Work out the finished part from the listing and answer in its coordinate system (mm). Face numbers are marked on the shaded views. A direction names the side the tool comes from. Coordinates: 2 decimals unless noted, no trailing zeros. Order: outer loops, then holes, each group sorted by start corner. A loop starts at its lowest first (then second) coordinate and runs counter-clockwise, first axis right, second up. Notation, with made-up numbers: M -40,67 L -8,67 A20 cw -8,93 Z; hole C 75,-4.75 d7. An arc over 180 degrees is marked long. Use a Markdown table: item, result.
from build123d import *

# Parameters (mm, degrees)
BOSS_EXTRUDE1_DEPTH   = 30
CUT_EXTRUDE1_DEPTH    = 5
FILLET1_R             = 5
CHAMFER1_SIZE         = 1
M3X0_5_TAPPED_HOLE1_D = 2.5


with BuildPart() as part:
    # Sketch1 → Boss-Extrude1 (new, symmetric)
    with BuildSketch(Plane(origin=(0, 0, 0), x_dir=(0, 0, -1), z_dir=(1, 0, 0))):
        Polygon((-17.5, 10), (17.5, 10), (17.5, 0), (4, 0), (4, -3), (-4, -3), (-4, 0), (-17.5, 0), align=None)
    extrude(amount=BOSS_EXTRUDE1_DEPTH, both=True)

    # Sketch3 → CSK for M6 Flat Head Machine Screw1 (revolve, cut)
    with BuildSketch(Plane(origin=(0, 10, 0), x_dir=(0, 0, 1), z_dir=(1, 0, 0))):
        Polygon((0, 0), (0, 13), (3.3, 13), (3.3, 8), (6.3, 5), (6.3, 0), align=None)
    revolve(axis=Axis((0, 16.35, 0), (0, -1, 0)), mode=Mode.SUBTRACT)

    # Sketch4 → Cut-Extrude1 (cut, symmetric)
    with BuildSketch(Plane(origin=(20, 0, 0), x_dir=(0, 0, -1), z_dir=(1, 0, 0))):
        with BuildLine():
            Line((-15, 10), (-10, 10))
            ThreePointArc((-10, 10), (-7.5, 7.5), (-5, 10))
            Line((-5, 10), (0, 10))
            ThreePointArc((0, 10), (-7.5, 2.5), (-15, 10))
        make_face()
    cut_extrude1 = extrude(amount=CUT_EXTRUDE1_DEPTH, both=True, mode=Mode.SUBTRACT)

    # Mirror1: Cut-Extrude1 across plane
    add(cut_extrude1.mirror(Plane(origin=(0, 0, 0), x_dir=(0, 0, 1), z_dir=(1, 0, 0))), mode=Mode.SUBTRACT)

    # Fillet1
    fillet1_edges = [part.edges().sort_by_distance(p)[0] for p in [
        (-30, 5, 17.5),
        (30, 5, -17.5),
        (30, 5, 17.5),
        (-30, 5, -17.5),
    ]]
    fillet(fillet1_edges, radius=FILLET1_R)

    # Chamfer1
    # the kernel refuses this chamfer: 1 mm, written as the material it takes off along each edge
    with BuildSketch(Plane(origin=(-30, -5.571682988, 4), x_dir=(-0.027495876610585623, 0, -0.9996219169112968), z_dir=(0, 1, 0)), Plane(origin=(-30, 0, -4), x_dir=(-0.027495876610585623, 0, 0.9996219169112968), z_dir=(0, -1, 0))) as chamfer1_piece_1:
        Polygon((CHAMFER1_SIZE * 0.999621916911, -CHAMFER1_SIZE * 0.0274958766106), (-CHAMFER1_SIZE * 0.0274958766106, -CHAMFER1_SIZE * 0.999621916911), (0, 0), align=None)
    extrude(amount=5.571682988, mode=Mode.SUBTRACT)
    with BuildSketch(Plane(origin=(30, -5.571682988, 4), x_dir=(0.027495876610585623, 0, -0.9996219169112968), z_dir=(0, 1, 0)), Plane(origin=(30, 0, -4), x_dir=(0.027495876610585623, 0, 0.9996219169112968), z_dir=(0, -1, 0))) as chamfer1_piece_2:
        Polygon((CHAMFER1_SIZE * 0.999621916911, CHAMFER1_SIZE * 0.0274958766106), (-CHAMFER1_SIZE * 0.0274958766106, CHAMFER1_SIZE * 0.999621916911), (0, 0), align=None)
    extrude(amount=5.571682988, mode=Mode.SUBTRACT)
    with BuildSketch(Plane(origin=(32.571682988, -3, -4), x_dir=(0, 0.9996219169112968, -0.027495876610586494), z_dir=(-1, 0, 0))) as chamfer1_piece_3:
        Polygon((CHAMFER1_SIZE * 0.999621916911, -CHAMFER1_SIZE * 0.0274958766106), (-CHAMFER1_SIZE * 0.0274958766106, -CHAMFER1_SIZE * 0.999621916911), (0, 0), align=None)
    extrude(amount=65.143365976, mode=Mode.SUBTRACT)
    with BuildSketch(Plane(origin=(32.571682988, -3, 4), x_dir=(0, 0.9996219169112968, 0.027495876610586494), z_dir=(-1, 0, 0))) as chamfer1_piece_4:
        Polygon((CHAMFER1_SIZE * 0.999621916911, CHAMFER1_SIZE * 0.0274958766106), (-CHAMFER1_SIZE * 0.0274958766106, CHAMFER1_SIZE * 0.999621916911), (0, 0), align=None)
    extrude(amount=65.143365976, mode=Mode.SUBTRACT)
    with BuildSketch(Plane(origin=(30, 0, -12.5), x_dir=(0.027495876610585623, 0.9996219169112968, 0), z_dir=(0, 0, 1)), Plane(origin=(30, 0, 4), x_dir=(0.02749587661058563, 0.9996219169112968, 0), z_dir=(0, 0, 1))) as chamfer1_piece_5:
        Polygon((CHAMFER1_SIZE * 0.999621916911, CHAMFER1_SIZE * 0.0274958766106), (-CHAMFER1_SIZE * 0.0274958766106, CHAMFER1_SIZE * 0.999621916911), (0, 0), align=None)
    extrude(amount=8.5, mode=Mode.SUBTRACT)
    with BuildSketch(Plane(origin=(-30, 0, 4), x_dir=(-0.02749587661058563, 0.9996219169112968, 0), z_dir=(0, 0, 1)), Plane(origin=(-30, 0, -12.5), x_dir=(-0.027495876610585623, 0.9996219169112968, 0), z_dir=(0, 0, 1))) as chamfer1_piece_6:
        Polygon((CHAMFER1_SIZE * 0.999621916911, -CHAMFER1_SIZE * 0.0274958766106), (-CHAMFER1_SIZE * 0.0274958766106, -CHAMFER1_SIZE * 0.999621916911), (0, 0), align=None)
    extrude(amount=8.5, mode=Mode.SUBTRACT)
    with BuildSketch(Plane(origin=(-25, 0, 17.5), x_dir=(0, 0.9996219169112968, 0.02749587661058563), z_dir=(1, 0, 0)), Plane(origin=(25, 0, -17.5), x_dir=(0, 0.9996219169112968, -0.027495876610585623), z_dir=(-1, 0, 0))) as chamfer1_piece_7:
        Polygon((CHAMFER1_SIZE * 0.999621916911, -CHAMFER1_SIZE * 0.0274958766106), (-CHAMFER1_SIZE * 0.0274958766106, -CHAMFER1_SIZE * 0.999621916911), (0, 0), align=None)
    extrude(amount=50, mode=Mode.SUBTRACT)
    with BuildSketch(Plane(origin=(-25, 0, 12.5), x_dir=(0, 0, 1), z_dir=(1, 0, 0))) as chamfer1_piece_8:
        Polygon((5, -CHAMFER1_SIZE), (5 - CHAMFER1_SIZE, 0), (5, 0), align=None)
    revolve(axis=Axis((-25, 0, 12.5), (0, -1, 0)), revolution_arc=90, mode=Mode.SUBTRACT)
    with BuildSketch(Plane(origin=(25, 0, 12.5), x_dir=(0, 0, 1), z_dir=(-1, 0, 0))) as chamfer1_piece_9:
        Polygon((5, CHAMFER1_SIZE), (5 - CHAMFER1_SIZE, 0), (5, 0), align=None)
    revolve(axis=Axis((25, 0, 12.5), (0, 1, 0)), revolution_arc=90, mode=Mode.SUBTRACT)
    with BuildSketch(Plane(origin=(-25, 0, -12.5), x_dir=(-1, 0, 0), z_dir=(0, 0, 1))) as chamfer1_piece_10:
        Polygon((5, -CHAMFER1_SIZE), (5 - CHAMFER1_SIZE, 0), (5, 0), align=None)
    revolve(axis=Axis((-25, 0, -12.5), (0, -1, 0)), revolution_arc=90, mode=Mode.SUBTRACT)
    with BuildSketch(Plane(origin=(25, 0, -12.5), x_dir=(1, 0, 0), z_dir=(0, 0, 1))) as chamfer1_piece_11:
        Polygon((5, CHAMFER1_SIZE), (5 - CHAMFER1_SIZE, 0), (5, 0), align=None)
    revolve(axis=Axis((25, 0, -12.5), (0, 1, 0)), revolution_arc=90, mode=Mode.SUBTRACT)
    with BuildSketch(Plane(origin=(-30, 0, 1.428317012), x_dir=(-0.02749587661058563, 0.9996219169112968, 0), z_dir=(0, 0, 1))) as chamfer1_piece_12a_section:
        Polygon((CHAMFER1_SIZE * 0.999621916911, -CHAMFER1_SIZE * 0.0274958766106), (-CHAMFER1_SIZE * 0.0274958766106, -CHAMFER1_SIZE * 0.999621916911), (0, 0), align=None)
    chamfer1_piece_12a = extrude(amount=11.071682988, mode=Mode.PRIVATE)
    chamfer1_piece_12a = split(chamfer1_piece_12a, bisect_by=Plane(origin=(-29.670206373, 0.329793627, 4), z_dir=(0, 0, -1)), keep=Keep.TOP, mode=Mode.PRIVATE)
    with BuildSketch(Plane(origin=(-30, -5.571682988, 4), x_dir=(-0.027495876610585623, 0, -0.9996219169112968), z_dir=(0, 1, 0))) as chamfer1_piece_12b_section:
        Polygon((CHAMFER1_SIZE * 0.999621916911, -CHAMFER1_SIZE * 0.0274958766106), (-CHAMFER1_SIZE * 0.0274958766106, -CHAMFER1_SIZE * 0.999621916911), (0, 0), align=None)
    chamfer1_piece_12b = extrude(amount=8.143365976, mode=Mode.PRIVATE)
    chamfer1_piece_12b = split(chamfer1_piece_12b, bisect_by=Plane(origin=(-29.670206373, 0, 3.670206373), z_dir=(0, 1, 0)), keep=Keep.TOP, mode=Mode.PRIVATE)
    chamfer1_piece_12 = chamfer1_piece_12a & chamfer1_piece_12b
    add(chamfer1_piece_12, mode=Mode.SUBTRACT)
    with BuildSketch(Plane(origin=(30, 0, 1.428317012), x_dir=(0.02749587661058563, 0.9996219169112968, 0), z_dir=(0, 0, 1))) as chamfer1_piece_13a_section:
        Polygon((CHAMFER1_SIZE * 0.999621916911, CHAMFER1_SIZE * 0.0274958766106), (-CHAMFER1_SIZE * 0.0274958766106, CHAMFER1_SIZE * 0.999621916911), (0, 0), align=None)
    chamfer1_piece_13a = extrude(amount=11.071682988, mode=Mode.PRIVATE)
    chamfer1_piece_13a = split(chamfer1_piece_13a, bisect_by=Plane(origin=(29.670206373, 0.329793627, 4), z_dir=(0, 0, -1)), keep=Keep.TOP, mode=Mode.PRIVATE)
    with BuildSketch(Plane(origin=(30, -5.571682988, 4), x_dir=(0.027495876610585623, 0, -0.9996219169112968), z_dir=(0, 1, 0))) as chamfer1_piece_13b_section:
        Polygon((CHAMFER1_SIZE * 0.999621916911, CHAMFER1_SIZE * 0.0274958766106), (-CHAMFER1_SIZE * 0.0274958766106, CHAMFER1_SIZE * 0.999621916911), (0, 0), align=None)
    chamfer1_piece_13b = extrude(amount=8.143365976, mode=Mode.PRIVATE)
    chamfer1_piece_13b = split(chamfer1_piece_13b, bisect_by=Plane(origin=(29.670206373, 0, 3.670206373), z_dir=(0, 1, 0)), keep=Keep.TOP, mode=Mode.PRIVATE)
    chamfer1_piece_13 = chamfer1_piece_13a & chamfer1_piece_13b
    add(chamfer1_piece_13, mode=Mode.SUBTRACT)
    with BuildSketch(Plane(origin=(30, 0, -12.5), x_dir=(0.027495876610585623, 0.9996219169112968, 0), z_dir=(0, 0, 1))) as chamfer1_piece_14a_section:
        Polygon((CHAMFER1_SIZE * 0.999621916911, CHAMFER1_SIZE * 0.0274958766106), (-CHAMFER1_SIZE * 0.0274958766106, CHAMFER1_SIZE * 0.999621916911), (0, 0), align=None)
    chamfer1_piece_14a = extrude(amount=11.071682988, mode=Mode.PRIVATE)
    chamfer1_piece_14a = split(chamfer1_piece_14a, bisect_by=Plane(origin=(29.670206373, 0.329793627, -4), z_dir=(0, 0, 1)), keep=Keep.TOP, mode=Mode.PRIVATE)
    with BuildSketch(Plane(origin=(30, 2.571682988, -4), x_dir=(0.027495876610585623, 0, 0.9996219169112968), z_dir=(0, -1, 0))) as chamfer1_piece_14b_section:
        Polygon((CHAMFER1_SIZE * 0.999621916911, CHAMFER1_SIZE * 0.0274958766106), (-CHAMFER1_SIZE * 0.0274958766106, CHAMFER1_SIZE * 0.999621916911), (0, 0), align=None)
    chamfer1_piece_14b = extrude(amount=8.143365976, mode=Mode.PRIVATE)
    chamfer1_piece_14b = split(chamfer1_piece_14b, bisect_by=Plane(origin=(29.670206373, 0, -3.670206373), z_dir=(0, 1, 0)), keep=Keep.TOP, mode=Mode.PRIVATE)
    chamfer1_piece_14 = chamfer1_piece_14a & chamfer1_piece_14b
    add(chamfer1_piece_14, mode=Mode.SUBTRACT)
    with BuildSketch(Plane(origin=(-30, 0, -12.5), x_dir=(-0.027495876610585623, 0.9996219169112968, 0), z_dir=(0, 0, 1))) as chamfer1_piece_15a_section:
        Polygon((CHAMFER1_SIZE * 0.999621916911, -CHAMFER1_SIZE * 0.0274958766106), (-CHAMFER1_SIZE * 0.0274958766106, -CHAMFER1_SIZE * 0.999621916911), (0, 0), align=None)
    chamfer1_piece_15a = extrude(amount=11.071682988, mode=Mode.PRIVATE)
    chamfer1_piece_15a = split(chamfer1_piece_15a, bisect_by=Plane(origin=(-29.670206373, 0.329793627, -4), z_dir=(0, 0, 1)), keep=Keep.TOP, mode=Mode.PRIVATE)
    with BuildSketch(Plane(origin=(-30, 2.571682988, -4), x_dir=(-0.027495876610585623, 0, 0.9996219169112968), z_dir=(0, -1, 0))) as chamfer1_piece_15b_section:
        Polygon((CHAMFER1_SIZE * 0.999621916911, -CHAMFER1_SIZE * 0.0274958766106), (-CHAMFER1_SIZE * 0.0274958766106, -CHAMFER1_SIZE * 0.999621916911), (0, 0), align=None)
    chamfer1_piece_15b = extrude(amount=8.143365976, mode=Mode.PRIVATE)
    chamfer1_piece_15b = split(chamfer1_piece_15b, bisect_by=Plane(origin=(-29.670206373, 0, -3.670206373), z_dir=(0, 1, 0)), keep=Keep.TOP, mode=Mode.PRIVATE)
    chamfer1_piece_15 = chamfer1_piece_15a & chamfer1_piece_15b
    add(chamfer1_piece_15, mode=Mode.SUBTRACT)

    # M3x0.5 Tapped Hole1 (through all)
    with Locations(Plane(origin=(0, 10, 0), x_dir=(1, 0, 0), z_dir=(0, 1, 0))):
        with Locations((-9.5, 13), (9.5, 13)):
            Hole(M3X0_5_TAPPED_HOLE1_D / 2)


solid = part.part
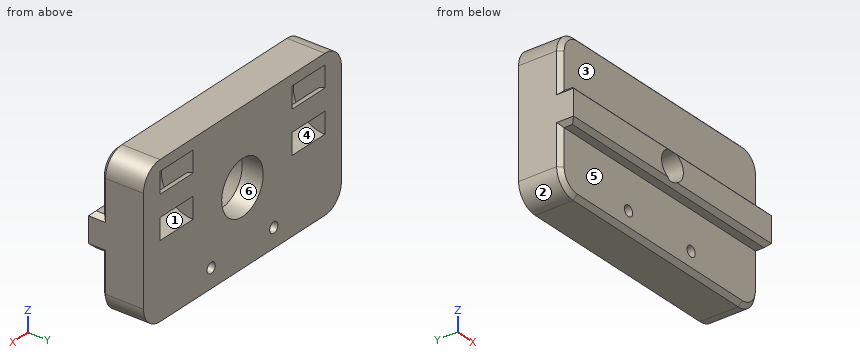
1. For the marked faces 4, 5 and 6, determine the directions among +Z, -Z, +X, -X, +Y, -Y from which every point of the face is accessible in a straight line to the end or side of a thin tool.
Answers below:
| item | result |
|---|---|
| face 4 | none |
| face 5 | -Z, +X, -X, -Y |
| face 6 | +Y |
2. Section A-A on x = 0 is taken. Determine the outline of the cut face in (y, z), then the cut area to 3 significant figures.
Answers below:
| item | result |
|---|---|
| outline | M -2.7,-3.3 L -2,-4 L 0,-4 L 0,-16.5 L 1,-17.5 L 10,-17.5 L 10,-6.3 L 5,-6.3 L 2,-3.3 Z; M -2.7,3.3 L 2,3.3 L 5,6.3 L 10,6.3 L 10,17.5 L 1,17.5 L 0,16.5 L 0,4 L -2,4 Z |
| area | 247 mm² |
3. For a pull along X with two mould halves and no side action, classify the marked faces 1, 2 and 3 as +X half, -X half, draft (parallel to the pull), parting line (faces both ways), or undercut.
Answers below:
| item | result |
|---|---|
| face 1 | undercut |
| face 2 | -X half |
| face 3 | draft |
4. Flat-ended cylindrical pins translate along their axes: P1, Ø10, axis at x = -8.5, z = -11.5, coming from the -Y side; P2, Ø1.6, axis at x = -3, y = -0.5, coming from the -Z side; P3, Ø1.5, axis at y = 3.5, z = 13.5, coming from the +X side. Find the tip coordinate at first contact, or state that the pin passes through.
Answers below:
| item | result |
|---|---|
| P1 | y = 0 |
| P2 | z = -16.8 |
| P3 | x = 29.99 |
5. Section D-D on x = 7 is taken. Determine the outline of the cut face in (y, z).
Answers below:
| item | result |
|---|---|
| outline | M -3,-3 L -2,-4 L 0,-4 L 0,-16.5 L 1,-17.5 L 10,-17.5 L 10,17.5 L 1,17.5 L 0,16.5 L 0,4 L -2,4 L -3,3 Z |
6. Section B-B on z = 7.5 is taken. Determine the outline of the cut face in (x, y).
Answers below:
| item | result |
|---|---|
| outline | M -30,1 L -29,0 L 29,0 L 30,1 L 30,10 L -30,10 Z; hole M -25,2.5 L -15,2.5 L -15,7.5 L -25,7.5 Z; hole M 15,2.5 L 25,2.5 L 25,7.5 L 15,7.5 Z |
7. Section C-C on y = -1.25 is taken. Determine the outline of the cut face in (x, z), then the cut area to 3 significant figures.
Answers below:
| item | result |
|---|---|
| outline | M -30,-3 L -29,-4 L 29,-4 L 30,-3 L 30,3 L 29,4 L -29,4 L -30,3 Z; hole C 0,0 d6.6 |
| area | 444 mm² |
8. Find the intervals of material crossed by probe 1 along X at (y, z) = (3.25, 5); probe 2 along X at (y, z) = (-0.3, 0); probe 3 along X at (y, z) = (2.75, -13), in increasing order.
Answers below:
| item | result |
|---|---|
| probe 1 | -30 to -25, -15 to 15, 25 to 30 |
| probe 2 | -30 to -3.3, 3.3 to 30 |
| probe 3 | -29.97 to -10.75, -8.25 to 8.25, 10.75 to 29.97 |
